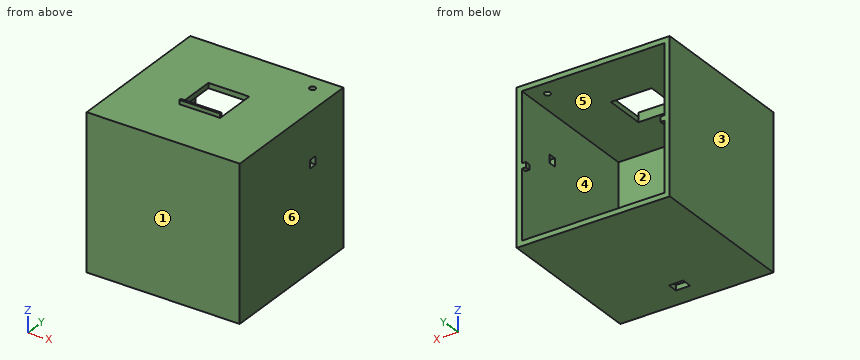
Autodesk Inventor part; units mm, degrees
ref_plane "YZ Plane" through (0, 0, 0) normal (1, 0, 0) x (0, 1, 0)
ref_plane "XZ Plane" through (0, 0, 0) normal (0, 1, 0) x (-1, 0, 0)
ref_plane "XY Plane" through (0, 0, 0) normal (0, 0, 1) x (1, 0, 0)
sketch "Náčrt1" plane through (0, 0, 0) normal (0, 0, 1) x (1, 0, 0)
  line L0 (0, 105) -> (0, -105)
  line L1 (-105, 0) -> (105, 0)
  line L2 (-75, 75) -> (75, 75)
  line L3 (75, 75) -> (75, -75)
  line L4 (75, -75) -> (-75, -75)
  line L5 (-75, -75) -> (-75, 75)
  point P0 (0, 0)
  dimension "d0" = 150
  dimension "d1" = 150
extrude "Vysunutí1" add sketch "Náčrt1" along normal blind 150
sketch "Náčrt2" plane through (-75, 75, 0) normal (0, 1, 0) x (1, 0, 0)
  line L0 (0, 0) -> (0, -150)
  line L1 (150, 0) -> (0, 0)
  line L2 (5, -145) -> (145, -145)
  line L3 (145, -145) -> (145, -5)
  line L4 (145, -5) -> (5, -5)
  line L5 (5, -5) -> (5, -145)
  point P0 (75, 0)
  dimension "d4" = 140
  dimension "d5" = 140
  dimension "d6" = 5
  dimension "d7" = 5
extrude "Vysunutí2" cut sketch "Náčrt2" against normal blind 140
sketch "Náčrt3" plane through (0, 0, 150) normal (0, 0, 1) x (1, 0, 0)
  line L0 (-20, 20) -> (20, 20)
  line L1 (20, 20) -> (20, -20)
  line L2 (20, -20) -> (-20, -20)
  line L3 (-20, -20) -> (-20, 20)
  line L4 (0, 105) -> (0, -105)
  line L5 (-105, 0) -> (105, 0)
  line L6 (-75, -75) -> (75, -75)
  circle A0 centre (55, 60) radius 3
  line L7 (75, -75) -> (75, 75)
  line L8 (75, 75) -> (-75, 75)
  point P0 (0, 0)
  dimension "d10" = 40
  dimension "d11" = 40
  dimension "d12" = 55
  dimension "d13" = 6
  dimension "d14" = 20
  dimension "d15" = 15
extrude "Vysunutí3" cut sketch "Náčrt3" against normal blind 10 contours L0 L4 L5 L3 | L0 L1 L5 L4 | L5 L4 L2 L3 | L5 L1 L2 L4 | A0
sketch "Náčrt36" plane through (75, -75, 0) normal (1, 0, 0) x (0, 0, -1)
  line L0 (-105, 110) -> (-97, 110)
  line L1 (-97, 110) -> (-97, 102)
  line L2 (-97, 102) -> (-105, 102)
  line L3 (-105, 102) -> (-105, 110)
  line L4 (0, 0) -> (0, 150)
  line L5 (0, 150) -> (-150, 150)
  line L6 (-150, 0) -> (-150, 150)
  line L7 (0, 0) -> (-150, 0)
  point P0 (0, 75)
  dimension "d188" = 8
  dimension "d189" = 8
  dimension "d190" = 40
  dimension "d191" = 45
extrude "Vysunutí28" cut sketch "Náčrt36" against normal blind 10 contours L0 L1 L2 L3
sketch "Náčrt37" plane through (0, 0, 150) normal (0, 0, 1) x (1, 0, 0)
  line L0 (-20, -20) -> (-20, 20)
  line L1 (-20, -20) -> (20, -20)
  line L2 (20, -20) -> (20, -22)
  line L3 (20, -22) -> (-20, -22)
  line L4 (-20, -22) -> (-20, -20)
  point P0 (0, 0)
  dimension "d194" = 2
  dimension "d195" = 40
extrude "Vysunutí29" add sketch "Náčrt37" along normal blind 4
sketch "Náčrt38" plane through (-70, 75, 145) normal (1, 0, 0) x (0, 0, -1)
  line L0 (0, 0) -> (140, 0)
  line L1 (0, 0) -> (0, -140)
  line L2 (0, -140) -> (140, -140)
  line L3 (140, 0) -> (140, -140)
  line L4 (67.5, 0) -> (72.5, 0)
  line L5 (72.5, 0) -> (72.5, -5)
  line L6 (72.5, -5) -> (67.5, -5)
  line L7 (67.5, -5) -> (67.5, 0)
  point P0 (145, -75)
  dimension "d198" = 5
  dimension "d199" = 5
  dimension "d200" = 67.5
extrude "Vysunutí30" add sketch "Náčrt38" along normal blind 4 contours L0 L5 L6 L7
sketch "Náčrt39" plane through (70, 75, 5) normal (-1, 0, 0) x (0, 0, 1)
  line L0 (92, -48) -> (92, -40)
  line L1 (92, -40) -> (100, -40)
  line L2 (100, -40) -> (100, -48)
  line L3 (100, -48) -> (92, -48)
  line L4 (0, 0) -> (140, 0)
  line L5 (0, 0) -> (0, -140)
  line L6 (0, -140) -> (140, -140)
  line L7 (140, 0) -> (140, -140)
  line L8 (67.5, 0) -> (72.5, 0)
  line L9 (72.5, 0) -> (72.5, -5)
  line L10 (72.5, -5) -> (67.5, -5)
  line L11 (67.5, -5) -> (67.5, 0)
  point P0 (-5, -75)
  point P1 (72.5, 0)
  dimension "d203" = 5
  dimension "d204" = 5
  dimension "d205" = 67.5
extrude "Vysunutí31" add sketch "Náčrt39" along normal blind 4 contours L4 L9 L10 L11
sketch "Náčrt41" plane through (0, 0, 0) normal (0, 0, -1) x (-1, 0, 0)
  line L0 (75, -75) -> (-75, -75)
  line L1 (75, 75) -> (75, -75)
  line L2 (-75, 75) -> (75, 75)
  line L3 (-75, -75) -> (-75, 75)
  line L4 (-7, -45) -> (7, -45)
  line L5 (7, -45) -> (7, -55)
  line L6 (7, -55) -> (-7, -55)
  line L7 (-7, -55) -> (-7, -45)
  line L8 (0, -105) -> (0, 105)
  point P0 (0, 0)
  dimension "d209" = 14
  dimension "d210" = 10
  dimension "d211" = 20
extrude "Vysunutí32" cut sketch "Náčrt41" against normal blind 10 contours L8 L4 L5 L6 | L6 L7 L4 L8
properties part number "Box na elektro"
Verification items for the finished model (mm, model axes). Face numbers are marked on the shaded views. A direction names the side the tool comes from. Round coordinates to 2 decimals unless told otherwise and drop trailing zeros. Write each loop counter-clockwise with the first axis right and the second up, starting at its lowest first coordinate (ties: lowest second). Pieces come first, ordered by that corner, then holes.
1. Scan lines: L1, parallel to Z at x = 55, y = 17.5; L2, parallel to Y at x = 55, z = 148.5; L3, parallel to X at y = -40.5, z = 53. Record each from-to range of solid material in increasing order.
2. Section check B-B on y = 13. Enter the section's corners in (x, z).
3. Draft check along X on the marked faces 1, 2, 3 and 4. Enter one of: +X half, -X half, draft (parallel to the pull), parting line (faces both ways), or undercut.
4. Section check C-C on x = 55. Enter the section's corners in (y, z), plus the area to 3 significant figures.
5. Access from +Z, -Z, +X, -X, +Y, -Y to the whole of each face (thin tool, end or side, straight path). Record for the marked faces 5 and 6.
6. Section check D-D on z = 134. Enter the section's corners in (x, y).
7. Section check A-A on x = 3. Enter the section's corners in (y, z), plus the area to 3 significant figures.
8. Gauge pin test, flat ends, axial feed: P1, Ø4.5, axis at x = -9.5, z = 152.5, coming from the -Y side; P2, Ø1, axis at y = -21, z = 152.5, coming from the -X side; P3, Ø8, axis at x = 2, z = 56.5, coming from the +Y side. Record the tip position at first contact, or that the pin passes through.
Answer:
1. L1: z = 0 to 5, 145 to 150
1. L2: y = -75 to 57, 63 to 75
1. L3: x = -75 to -70, 70 to 75
2. outline: (-75, 0) - (75, 0) - (75, 150) - (20, 150) - (20, 145) - (70, 145) - (70, 5) - (-70, 5) - (-70, 145) - (-20, 145) - (-20, 150) - (-75, 150) - close
3. face 1: draft
3. face 2: undercut
3. face 3: -X half
3. face 4: undercut
4. outline: (-75, 0) - (75, 0) - (75, 5) - (-65, 5) - (-65, 145) - (57, 145) - (57, 150) - (-75, 150) - close; (63, 145) - (75, 145) - (75, 150) - (63, 150) - close
4. area: 2,870 mm2
5. face 5: +Y
5. face 6: +Z, -Z, +X, +Y, -Y
6. outline: (-75, -75) - (75, -75) - (75, 75) - (70, 75) - (70, -65) - (-70, -65) - (-70, 75) - (-75, 75) - close
7. outline: (-75, 0) - (-55, 0) - (-55, 5) - (-65, 5) - (-65, 145) - (-20, 145) - (-20, 154) - (-22, 154) - (-22, 150) - (-75, 150) - close; (-45, 0) - (75, 0) - (75, 5) - (-45, 5) - close; (20, 145) - (75, 145) - (75, 150) - (20, 150) - close
7. area: 2,660 mm2
8. P1: stops at y = -22
8. P2: stops at x = -20
8. P3: stops at y = -65
